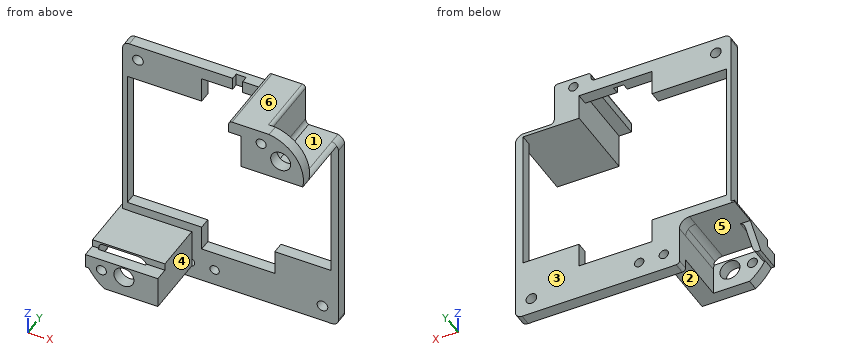
from build123d import *

# Parameters (mm, degrees)
SKETCH2_R           = 1.4
SKETCH2_R_2         = 1.6
BOSS_EXTRUDE1_DEPTH = 3.5
SKETCH3_R           = 1.4
BOSS_EXTRUDE2_DEPTH = 15.8
SKETCH4_R           = 3
SKETCH4_R_2         = 1.5
BOSS_EXTRUDE3_DEPTH = 3.5
SKETCH5_W           = 3
SKETCH5_H           = 3.708496363
BOSS_EXTRUDE4_DEPTH = 1.5
SKETCH7_W           = 35.498397003
SKETCH7_H           = 12.144188448
CUT_EXTRUDE2_DEPTH  = 4
BOSS_EXTRUDE5_DEPTH = 1
SKETCH6_W           = 15.172785082
SKETCH6_H           = 14.006435155
CUT_EXTRUDE3_DEPTH  = 15
CHAMFER1_START      = -11.4
CHAMFER1_DEPTH      = 0.087265638
CHAMFER1_START_2    = -35.5
CHAMFER1_2_DEPTH    = 3
CHAMFER1_START_3    = -11.312734362
CHAMFER1_3_DEPTH    = 7.312734362


with BuildPart() as part:
    # Sketch2 → Boss-Extrude1 (new body)
    with BuildSketch(Plane.XZ.offset(-3.6)):
        with BuildLine():
            Line((11.111566046, -27.048023457), (11.111566046, -19.6))
            Line((11.111566046, -19.6), (27.9, -19.6))
            Line((27.9, -19.6), (27.9, 23.6))
            Line((27.9, 23.6), (11.111563156, 23.6))
            Line((11.111563156, 23.6), (11.111563156, 31.276925258))
            Line((11.111563156, 31.276925258), (1.5, 31.276925258))
            Line((1.5, 31.276925258), (1.5, 34.985421621))
            Line((1.5, 34.985421621), (6.463917188, 34.985421621))
            ThreePointArc((6.463917188, 34.985421621), (7.171023969, 35.278314839), (7.463917188, 35.985421621))
            Line((7.463917188, 35.985421621), (7.463917188, 36.75))
            ThreePointArc((7.463917188, 36.75), (7.756810407, 37.457106781), (8.463917188, 37.75))
            Line((8.463917188, 37.75), (17.5, 37.75))
            ThreePointArc((17.5, 37.75), (18.207106781, 37.457106781), (18.5, 36.75))
            Line((18.5, 36.75), (18.5, 26.25))
            ThreePointArc((18.5, 26.25), (18.73500033, 25.309374588), (19.384776166, 24.589796458))
            Line((19.384776166, 24.589796458), (28.192260407, 24.589796458))
            ThreePointArc((28.192260407, 24.589796458), (29.567455824, 23.740606822), (30.192257213, 22.25))
            Line((30.192257213, 22.25), (30.192257213, -35.750098385))
            ThreePointArc((30.192257213, -35.750098385), (29.606435992, -37.164248347), (28.192257213, -37.75))
            Line((28.192257213, -37.75), (-18, -37.75))
            ThreePointArc((-18, -37.75), (-18.707106781, -37.457106781), (-19, -36.75))
            Line((-19, -36.75), (-19, -25.75))
            ThreePointArc((-19, -25.75), (-19.878679656, -23.628679656), (-22, -22.75))
            Line((-22, -22.75), (-32.5, -22.75))
            ThreePointArc((-32.5, -22.75), (-33.207106781, -23.042893219), (-33.5, -23.75))
            Line((-33.5, -23.75), (-33.5, -27.662734362))
            ThreePointArc((-33.5, -27.662734362), (-33.792893219, -28.369841143), (-34.5, -28.662734362))
            Line((-34.5, -28.662734362), (-34.5, 32.985421621))
            ThreePointArc((-34.5, 32.985421621), (-33.914213562, 34.399635183), (-32.5, 34.985421621))
            Line((-32.5, 34.985421621), (-1.5, 34.985421621))
            Line((-1.5, 34.985421621), (-1.5, 31.276925258))
            Line((-1.5, 31.276925258), (-10.808436895, 31.276925258))
            Line((-10.808436895, 31.276925258), (-10.808436895, 23.6))
            Line((-10.808436895, 23.6), (-33.1, 23.6))
            Line((-33.1, 23.6), (-33.1, -19.6))
            Line((-33.1, -19.6), (-10.808436895, -19.6))
            Line((-10.808436895, -19.6), (-10.808436895, -27.048023457))
            Line((-10.808436895, -27.048023457), (11.111566046, -27.048023457))
        make_face()
        with Locations(Location((-6.918752516, -32.76626587, 0), (0, 0, 270))):
            Circle(SKETCH2_R, mode=Mode.SUBTRACT)
        with Locations(Location((25.4, -32.76626587, 0), (0, 0, 270))):
            Circle(SKETCH2_R_2, mode=Mode.SUBTRACT)
        with Locations(Location((-14.297096298, -32.76626587, 0), (0, 0, 270))):
            Circle(SKETCH2_R, mode=Mode.SUBTRACT)
        with Locations(Location((-29.911917882, 30.347920192, 0), (0, 0, 270))):
            Circle(SKETCH2_R_2, mode=Mode.SUBTRACT)
        with Locations(Location((12.814585658, 34.985421621, 0), (0, 0, 270))):
            Circle(SKETCH2_R, mode=Mode.SUBTRACT)
    extrude(amount=BOSS_EXTRUDE1_DEPTH)

    # Sketch3 → Boss-Extrude2 (add)
    # profile 1 of 2: a face of its own
    with BuildSketch(Plane(origin=(0, 0.1, 0), x_dir=(-1, 0, 0), z_dir=(0, -1, 0))):
        with BuildLine():
            Line((-7.463917188, -33.985421621), (-7.463917188, -36.75))
            ThreePointArc((-7.463917188, -36.75), (-7.756810407, -37.457106781), (-8.463917188, -37.75))
            Line((-8.463917188, -37.75), (-17.5, -37.75))
            ThreePointArc((-17.5, -37.75), (-18.207106781, -37.457106781), (-18.5, -36.75))
            Line((-18.5, -36.75), (-18.5, -26.25))
            ThreePointArc((-18.5, -26.25), (-18.73500033, -25.309374588), (-19.384776166, -24.589796458))
            Line((-19.384776166, -24.589796458), (-28.192260407, -24.589796458))
            ThreePointArc((-28.192260407, -24.589796458), (-29.052595302, -24.270206108), (-29.679602398, -23.6))
            Line((-29.679602398, -23.6), (-11.111563156, -23.6))
            Line((-11.111563156, -23.6), (-11.111563156, -24.25))
            Line((-11.111563156, -24.25), (-11.111563156, -33.985421621))
            Line((-11.111563156, -33.985421621), (-7.463917188, -33.985421621))
        make_face()
        with Locations(Location((-12.814585658, -34.985421621, 0), (0, 0, 90))):
            Circle(SKETCH3_R, mode=Mode.SUBTRACT)
    # profile 2 of 2: a face of its own
    with BuildSketch(Plane(origin=(0, 0.1, 0), x_dir=(-1, 0, 0), z_dir=(0, -1, 0))):
        with BuildLine():
            Line((13.774855788, 22.239537014), (34.5, 22.239537014))
            Line((34.5, 22.239537014), (34.5, 23.75))
            Line((34.5, 23.75), (34.5, 28.662734362))
            ThreePointArc((34.5, 28.662734362), (33.792893219, 28.369841143), (33.5, 27.662734362))
            Line((33.5, 27.662734362), (33.5, 23.75))
            ThreePointArc((33.5, 23.75), (33.207106781, 23.042893219), (32.5, 22.75))
            Line((32.5, 22.75), (22, 22.75))
            ThreePointArc((22, 22.75), (20.777489524, 23.010389054), (19.767197945, 23.746354576))
            ThreePointArc((19.767197945, 23.746354576), (19.198357074, 24.67724797), (19, 25.75))
            Line((19, 25.75), (19, 33.953406826))
            Line((19, 33.953406826), (13.774855788, 33.953406826))
            Line((13.774855788, 33.953406826), (13.774855788, 31.467318277))
            Line((13.774855788, 31.467318277), (13.774855788, 23.746354576))
            Line((13.774855788, 23.746354576), (13.774855788, 22.239537014))
        make_face()
    extrude(amount=BOSS_EXTRUDE2_DEPTH)

    # Sketch4 → Boss-Extrude3 (add)
    # profile 1 of 2: a face of its own
    with BuildSketch(Plane.XZ.offset(15.7)):
        with BuildLine():
            Line((11.111563156, 23.6), (29.679602398, 23.6))
            ThreePointArc((29.679602398, 23.6), (27.614927524, 32.806940788), (19.577713664, 37.75))
            Line((19.577713664, 37.75), (8.463917188, 37.75))
            ThreePointArc((8.463917188, 37.75), (7.756810407, 37.457106781), (7.463917188, 36.75))
            Line((7.463917188, 36.75), (7.463917188, 33.985421621))
            Line((7.463917188, 33.985421621), (11.111563156, 33.985421621))
            Line((11.111563156, 33.985421621), (11.111563156, 23.6))
        make_face()
        with Locations(Location((23.040610867, 29.824211278, 0), (0, 0, 270))):
            Circle(SKETCH4_R, mode=Mode.SUBTRACT)
        with Locations(Location((17.180435895, 33.650043419, 0), (0, 0, 28.392671192))):
            Circle(SKETCH4_R_2, mode=Mode.SUBTRACT)
    # profile 2 of 2: a face of its own
    with BuildSketch(Plane.XZ.offset(15.7)):
        with BuildLine():
            Line((-29.84427835, -33.953406826), (-13.774855788, -33.953406826))
            Line((-13.774855788, -33.953406826), (-13.774855788, -22.239537014))
            Line((-13.774855788, -22.239537014), (-34.5, -22.239537014))
            Line((-34.5, -22.239537014), (-34.5, -28.662734362))
            ThreePointArc((-34.5, -28.662734362), (-32.451529424, -31.553930311), (-29.84427835, -33.953406826))
        make_face()
        with Locations(Location((-23.956564477, -27.796810843, 0), (0, 0, 270))):
            Circle(SKETCH4_R, mode=Mode.SUBTRACT)
        with Locations(Location((-30.707720306, -27.953239531, 0), (0, 0, 270))):
            Circle(SKETCH4_R_2, mode=Mode.SUBTRACT)
    extrude(amount=BOSS_EXTRUDE3_DEPTH)

    # Sketch5 → Boss-Extrude4 (add)
    with BuildSketch(Plane(origin=(0, 3.6, 0), x_dir=(1, 0, 0), z_dir=(0, 1, 0))):
        with Locations((0, -33.13117344)):
            Rectangle(SKETCH5_W, SKETCH5_H)
    extrude(amount=-BOSS_EXTRUDE4_DEPTH)

    # Sketch7 → Cut-Extrude2 (cut)
    with BuildSketch(Plane.XZ.offset(19.2)):
        with Locations((-20.871227876, -18.320079155)):
            Rectangle(SKETCH7_W, SKETCH7_H)
    extrude(amount=-CUT_EXTRUDE2_DEPTH, mode=Mode.SUBTRACT)

    # Sketch8 → Boss-Extrude5 (add)
    with BuildSketch(Plane.ZY.offset(34.5)):
        Polygon((-24.392173379, -19.2), (-24.392173379, -15.2), (-22.239537014, -15.2), (-22.239537014, 0.1), (-22.239537014, 3.6), (-28.662734362, 3.6), (-28.662734362, -19.2), align=None)
    extrude(amount=BOSS_EXTRUDE5_DEPTH)

    # Sketch6 → Cut-Extrude3 (cut)
    with BuildSketch(Plane(origin=(0, 3.6, 0), x_dir=(1, 0, 0), z_dir=(0, 1, 0))):
        with Locations((-37.568827946, 29.753217578)):
            Rectangle(SKETCH6_W, SKETCH6_H)
    extrude(amount=-CUT_EXTRUDE3_DEPTH, mode=Mode.SUBTRACT)

    # Chamfer1: read off the stored shape, not the designer's step
    # Chamfer1 outline → Chamfer1 (add)
    with BuildSketch(Plane(origin=(0, 0, 0), x_dir=(1, 0, 0), z_dir=(0, 1, 0)).offset(CHAMFER1_START)):
        with BuildLine():
            Line((-33.5, 23.75), (-33.5, 27.662734362))
            ThreePointArc((-33.5, 27.662734362), (-33.792893219, 28.369841143), (-34.5, 28.662734362))
            Line((-34.5, 28.662734362), (-35.5, 28.662734362))
            Line((-35.5, 28.662734362), (-35.5, 22.75))
            Line((-35.5, 22.75), (-32.5, 22.75))
            ThreePointArc((-32.5, 22.75), (-33.207106781, 23.042893219), (-33.5, 23.75))
        make_face()
    extrude(amount=CHAMFER1_DEPTH)

    # Chamfer1 2 outline → Chamfer1 2 (add)
    with BuildSketch(Plane.YZ.offset(CHAMFER1_START_2)):
        Polygon((-11.312734362, -28.662734362), (-5.4, -22.75), (-11.312734362, -22.75), align=None)
    extrude(amount=CHAMFER1_2_DEPTH)

    # Chamfer1 3 outline → Chamfer1 3 (cut)
    with BuildSketch(Plane(origin=(0, 0, 0), x_dir=(1, 0, 0), z_dir=(0, 1, 0)).offset(CHAMFER1_START_3)):
        with BuildLine():
            ThreePointArc((-34.5, 28.662734362), (-33.792893219, 28.369841143), (-33.5, 27.662734362))
            Line((-33.5, 27.662734362), (-33.5, 23.75))
            ThreePointArc((-33.5, 23.75), (-33.207106781, 23.042893219), (-32.5, 22.75))
            Line((-32.5, 22.75), (-32.5, 30))
            Line((-32.5, 30), (-36, 30))
            Line((-36, 30), (-36, 28.662734363))
            Line((-36, 28.662734363), (-34.5, 28.662734362))
        make_face()
    extrude(amount=CHAMFER1_3_DEPTH, mode=Mode.SUBTRACT)


solid = part.part
Geometry: final body of the model. Coordinates: model frame, mm. Face numbers are marked on the shaded views. A direction names the side the tool comes from. Give positions to 0.01 mm unless a question says otherwise; leave off trailing zeros. Loops run counter-clockwise (first coordinate to the right, second up) from the corner with the lowest first, then second, coordinate; pieces in that order, holes last. Notation, with made-up numbers: M 65.5,36.5 L 96.5,36.5 A14 cw 96.5,60.5 Z; hole C -27.75,72 d6. An arc over 180 degrees is marked long. Put each result on its own line as item: value.
1) Cut plane A-A, the plane z = 14. Return the cut outline in (x, y).
Computed values:
outline: M -34.5,0.1 L -33.1,0.1 L -33.1,3.6 L -34.5,3.6 Z; M 27.9,0.1 L 30.19,0.1 L 30.19,3.6 L 27.9,3.6 Z
2) Reachability of the marked faces 1, 2 and 3 from +Z, -Z, +X, -X, +Y, -Y: full face, straight path, thin tool, end or side. Return the list, or none.
Computed values:
face 1: +Z, +X, +Y
face 2: -Z, +X, -X, -Y
face 3: +Z, -Z, +X, -X, +Y
3) Mould query, pull axis X, two halves, no side actions, for the marked faces 4, 5 and 6. Classes: released by +X, released by -X, zero draft, split by the parting line, or undercut.
Computed values:
face 4: released by +X
face 5: undercut
face 6: zero draft
4) Cut plane B-B, the plane x = 3.5. Return the cut outline in (y, z).
Computed values:
outline: M 0.1,-37.75 L 3.6,-37.75 L 3.6,-27.05 L 0.1,-27.05 Z; M 0.1,31.28 L 3.6,31.28 L 3.6,34.99 L 0.1,34.99 Z
5) First-contact query: P1, Ø3, axis at x = -27.5, y = -16.5, coming from the +Z side; P2, Ø9.5, axis at x = 23.04, z = 29.82, coming from the +Y side; P3, Ø1.4, axis at y = -10.5, z = 35, coming from the -X side; P4, Ø0.6, axis at x = -23, z = -23, coming from the -Y side. Flat tips, straight axial feed; report the tip coordinate or a pass-through.
Computed values:
P1: stops at z = -22.24
P2: stops at y = 3.6
P3: stops at x = 7.46
P4: stops at y = -15.2
6) Material intervals for L1, parallel to X at y = -9.75, z = 30.5; L2, parallel to Z at x = 17, y = -8.5; L3, parallel to X at y = -2.75, z = -22.5, sorted ascending. Write a range as from..to.
Computed values:
L1: x = 11.11..18.5
L2: z = 23.6..37.75
L3: x = -35.5..-13.77
7) Cut plane C-C, the plane y = -0.75. Return the cut outline in (x, z), plus the area to 3 significant figures.
Computed values:
outline: M -35.5,-22.75 L -22,-22.75 A3 cw -19,-25.75 L -19,-33.95 L -13.77,-33.95 L -13.77,-22.24 L -35.5,-22.24 Z; M 7.46,33.99 L 11.11,33.99 L 11.11,23.6 L 29.68,23.6 A2 ccw 28.19,24.59 L 19.38,24.59 A2 cw 18.5,26.25 L 18.5,36.75 A1 ccw 17.5,37.75 L 8.46,37.75 A1 ccw 7.46,36.75 Z; hole C 12.81,34.99 d2.8
area: 194 mm^2
